Part model, mm, in its own coordinate system. A direction names the side the tool comes from. Give positions to 0.01 mm unless a question says otherwise; leave off trailing zeros. Write each loop counter-clockwise with the first axis right and the second up, starting at its lowest first coordinate (ties: lowest second). Pieces come first, ordered by that corner, then holes. Notation, with made-up numbers: (-35.75, 10.5) - (-28.75, 10.5) arc R9 ccw to (-28.75, 14.5) - close; hole circle Ø7 at (13, -22.75). An arc over 180 degrees is marked (long way). Answer in a Markdown table with one row per item. Add a question column.
1. Band-saw the part on D-D on y = -21. Write the cut outline in (x, z).
2. Band-saw the part on B-B on x = 0. Write the cut outline in (y, z).
3. Band-saw the part on C-C on z = 3. Write the cut outline in (x, y), plus the area to 3 significant figures.
4. Probe line 1 along Y through (x, z) = (0, -14.05); line 2 along Z through (x, y) = (6, -69.5). List the from-to ranges inside material, lowest first.
5. Which spindle directions (+Z, -Z, +X, -X, +Y, -Y) get a long thin tool onto all of the face, cutting with end or side? Do faces 1 (the cylindrical face through (-0.62, -45.29, -13.93)), 2 (the flat face through (5, -47, -12.7)). Say none if no direction does.
6. Band-saw the part on A-A on y = -65. Write the cut outline in (x, z), plus the area to 4 significant figures.
7. Pull direction X, two halves, no side cores. Call faces 3 (the cylindrical face through (-1.03, -69.637, 13.968)), 4 (the flat face through (15.2, -47, 0)), 5 (the flat face through (-15.2, -47, 0)), 6 (the flat face through (-4, -47, 15.2)): released by +X, released by -X, zero draft, split by the parting line, or undercut.
```python
from build123d import *

# Parameters (mm, degrees)
F0_W     = 30.4
F0_H     = 30.4
F1_DEPTH = 95
F2_T     = -2.5
F3_R     = 4.75
F4_DEPTH = 38.5


with BuildPart() as f1:
    # F0 (on Front) → F1 (new body)
    with BuildSketch(Plane.XZ):
        Rectangle(F0_W, F0_H)
    extrude(amount=F1_DEPTH)

    # F2
    f2_openings = [f1.faces().sort_by_distance(p)[0] for p in [
        (0, -95, 0),
        (0, 0, 0),
    ]]
    offset(amount=F2_T, openings=f2_openings)

    # F3 (on face) → F4 (cut)
    with BuildSketch(Plane.XY.offset(15.2)):
        with Locations((0, -65)):
            Circle(F3_R)
        with Locations((0, -50)):
            Circle(F3_R)
    extrude(amount=-F4_DEPTH, mode=Mode.SUBTRACT)


solid = f1.part
```
Values:
| question | item | result |
|---|---|---|
| 1 | outline | (-15.2, -15.2) - (15.2, -15.2) - (15.2, 15.2) - (-15.2, 15.2) - close; hole (-12.7, -12.7) - (12.7, -12.7) - (12.7, 12.7) - (-12.7, 12.7) - close |
| 2 | outline | (-95, -15.2) - (-69.75, -15.2) - (-69.75, -12.7) - (-95, -12.7) - close; (-95, 12.7) - (-69.75, 12.7) - (-69.75, 15.2) - (-95, 15.2) - close; (-60.25, -15.2) - (-54.75, -15.2) - (-54.75, -12.7) - (-60.25, -12.7) - close; (-60.25, 12.7) - (-54.75, 12.7) - (-54.75, 15.2) - (-60.25, 15.2) - close; (-45.25, -15.2) - (0, -15.2) - (0, -12.7) - (-45.25, -12.7) - close; (-45.25, 12.7) - (0, 12.7) - (0, 15.2) - (-45.25, 15.2) - close |
| 3 | outline | (-15.2, -95) - (-12.7, -95) - (-12.7, 0) - (-15.2, 0) - close; (12.7, -95) - (15.2, -95) - (15.2, 0) - (12.7, 0) - close |
| 3 | area | 475 mm² |
| 4 | line 1 | y = -95 to -69.75, -60.25 to -54.75, -45.25 to 0 |
| 4 | line 2 | z = -15.2 to -12.7, 12.7 to 15.2 |
| 5 | face 1 | +Z, -Z |
| 5 | face 2 | +Y, -Y |
| 6 | outline | (-15.2, -15.2) - (-4.75, -15.2) - (-4.75, -12.7) - (-12.7, -12.7) - (-12.7, 12.7) - (-4.75, 12.7) - (-4.75, 15.2) - (-15.2, 15.2) - close; (4.75, -15.2) - (15.2, -15.2) - (15.2, 15.2) - (4.75, 15.2) - (4.75, 12.7) - (12.7, 12.7) - (12.7, -12.7) - (4.75, -12.7) - close |
| 6 | area | 231.5 mm² |
| 7 | face 3 | undercut |
| 7 | face 4 | released by +X |
| 7 | face 5 | released by -X |
| 7 | face 6 | zero draft |
